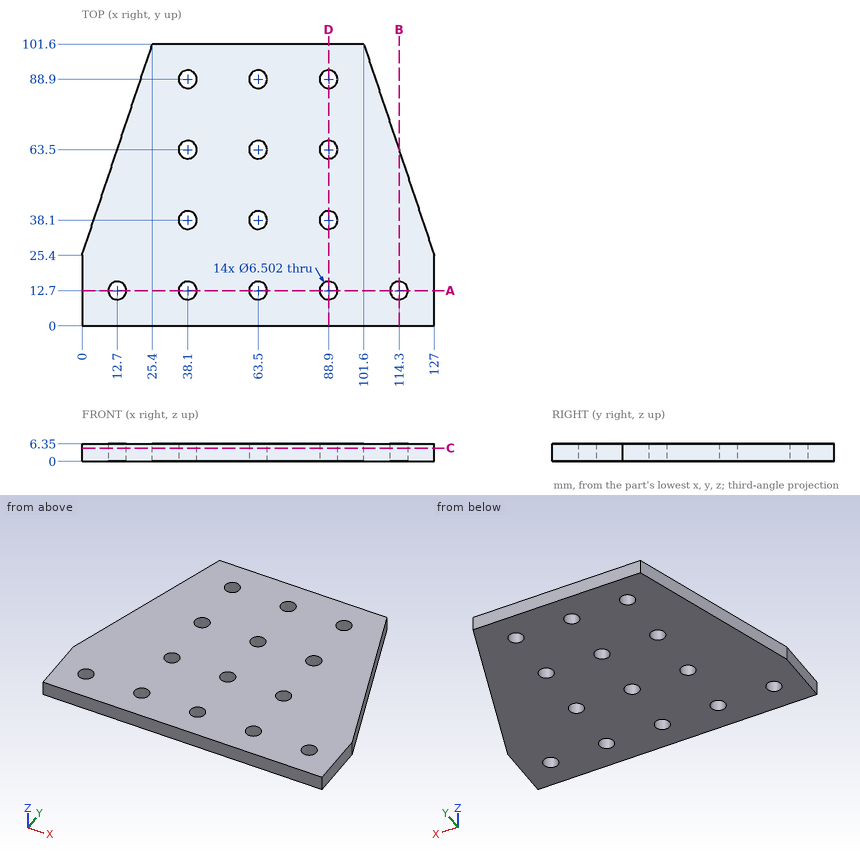
The drawing under review shows one solid part. Ordinate dimensions are in mm from its lowest x, y, z. Round coordinates to 2 decimals unless told otherwise and drop trailing zeros. Order: outer loops, then holes, each group sorted by start corner. A loop starts at its lowest first (then second) coordinate and runs counter-clockwise, first axis right, second up. Notation, with made-up numbers: (67.25, -11.75) -> (85.25, -11.75) arc R18 cw to (85.25, 14.25) -> close; hole circle Ø1 at (54, 63.5). An arc over 180 degrees is marked (long way). Use a Markdown table: item, result.
Item 1: Take a section at D-D (x = 88.9). State the section outline as (y, z) points.
Resolved:
| item | result |
|---|---|
| outline | (0, 0) -> (9.45, 0) -> (9.45, 6.35) -> (0, 6.35) -> close; (15.95, 0) -> (34.85, 0) -> (34.85, 6.35) -> (15.95, 6.35) -> close; (41.35, 0) -> (60.25, 0) -> (60.25, 6.35) -> (41.35, 6.35) -> close; (66.75, 0) -> (85.65, 0) -> (85.65, 6.35) -> (66.75, 6.35) -> close; (92.15, 0) -> (101.6, 0) -> (101.6, 6.35) -> (92.15, 6.35) -> close |
Item 2: Take a section at C-C (z = 4.75). State how many separate pieces and enclosed holes the cut face has, plus the area to 3 significant figures.
Resolved:
| item | result |
|---|---|
| separate pieces | 1 |
| enclosed holes | 14 |
| area | 10,500 mm² |
Item 3: For line 1 along Y through (x, z) = (38.1, 4.25); line 2 along X through (y, z) = (37, 1.5); line 3 along X through (y, z) = (61, 2.5) (1 decimal), list the stretches that pass through material, from the lowest coordinate up. Write a range as [from, to].
Resolved:
| item | result |
|---|---|
| line 1 | y = [0, 9.45], [15.95, 34.85], [41.35, 60.25], [66.75, 85.65], [92.15, 101.6] |
| line 2 | x = [3.87, 35.04], [41.16, 60.44], [66.56, 85.84], [91.96, 123.13] |
| line 3 | x = [11.9, 36], [40.2, 61.4], [65.6, 86.8], [91, 115.1] |
Item 4: Take a section at A-A (y = 12.7). State the section outline as (x, z) points, plus the area to 3 significant figures.
Resolved:
| item | result |
|---|---|
| outline | (0, 0) -> (9.45, 0) -> (9.45, 6.35) -> (0, 6.35) -> close; (15.95, 0) -> (34.85, 0) -> (34.85, 6.35) -> (15.95, 6.35) -> close; (41.35, 0) -> (60.25, 0) -> (60.25, 6.35) -> (41.35, 6.35) -> close; (66.75, 0) -> (85.65, 0) -> (85.65, 6.35) -> (66.75, 6.35) -> close; (92.15, 0) -> (111.05, 0) -> (111.05, 6.35) -> (92.15, 6.35) -> close; (117.55, 0) -> (127, 0) -> (127, 6.35) -> (117.55, 6.35) -> close |
| area | 600 mm² |
Item 5: Take a section at B-B (x = 114.3). State the section outline as (y, z) points.
Resolved:
| item | result |
|---|---|
| outline | (0, 0) -> (9.45, 0) -> (9.45, 6.35) -> (0, 6.35) -> close; (15.95, 0) -> (63.5, 0) -> (63.5, 6.35) -> (15.95, 6.35) -> close |
Item 6: For pin 1 (7.5 mm diameter, centred on x = 63.5, y = 12.7, fed in from -Z); pin 2 (6 mm diameter, centred on x = 88.9, y = 38.1, fed in from -Z); pin 3 (1 mm diameter, centred on y = 51, z = 5.5, fed in from -X), all flat-tipped, find the tip position at first contact; note any pin that passes through.
Resolved:
| item | result |
|---|---|
| pin 1 | stops at z = 0 |
| pin 2 | passes through |
| pin 3 | stops at x = 8.37 |
